Autodesk Inventor part; units mm, degrees
ref_plane "YZ Plane" through (0, 0, 0) normal (1, 0, 0) x (0, 1, 0)
ref_plane "XZ Plane" through (0, 0, 0) normal (0, 1, 0) x (-1, 0, 0)
ref_plane "XY Plane" through (0, 0, 0) normal (0, 0, 1) x (1, 0, 0)
sketch "Sketch1" plane through (0, 0, 0) normal (0, 0, 1) x (1, 0, 0)
  line L0 (0, 0) -> (25, 0)
  line L1 (25, 0) -> (25, 25)
  line L2 (25, 25) -> (0, 25)
  line L3 (0, 25) -> (0, 0)
  dimension "d0" = 25
  dimension "d1" = 25
extrude "Extrusion1" add sketch "Sketch1" along normal blind 2
sketch "Sketch2" plane through (0, 0, 2) normal (0, 0, 1) x (1, 0, 0)
  line L0 (0, 0) -> (0, 25)
  line L1 (0, 25) -> (25, 25)
  line L2 (2.5, 2.5) -> (22.5, 2.5)
  line L3 (22.5, 2.5) -> (22.5, 22.5)
  line L4 (22.5, 22.5) -> (2.5, 22.5)
  line L5 (2.5, 22.5) -> (2.5, 2.5)
  dimension "d4" = 20
  dimension "d5" = 20
  dimension "d6" = 2.5
  dimension "d7" = 2.5
extrude "Extrusion2" add sketch "Sketch2" along normal blind 3
sketch "Sketch3" plane through (0, 0, 0) normal (0, 0, -1) x (-1, 0, 0)
  line L0 (-25, 25) -> (0, 25)
  line L1 (-25, 0) -> (-25, 25)
  line L2 (-23.5, 23.5) -> (-1.5, 23.5)
  line L3 (-1.5, 23.5) -> (-1.5, 1.5)
  line L4 (-1.5, 1.5) -> (-23.5, 1.5)
  line L5 (-23.5, 1.5) -> (-23.5, 23.5)
  dimension "d10" = 22
  dimension "d11" = 22
  dimension "d12" = 1.5
  dimension "d13" = 1.5
extrude "Extrusion3" add sketch "Sketch3" along normal blind 3
properties part number "antena_gps"
Could you check a few things on this model? Use its own coordinates, in mm. A direction names the side the tool comes from. Round coordinates to 2 decimals unless told otherwise and drop trailing zeros. Write each loop counter-clockwise with the first axis right and the second up, starting at its lowest first coordinate (ties: lowest second). Pieces come first, ordered by that corner, then holes. Notation, with made-up numbers: (64, 74) - (79, 74) arc R18 cw to (79, 100) - close; hole circle Ø11 at (31.5, -21.5). An arc over 180 degrees is marked (long way). Use a Markdown table: item, result.
Q1. For pin 1 (1.5 mm diameter, centred on x = 9, z = 3.5, fed in from -Y); pin 2 (2.5 mm diameter, centred on x = 10.5, z = -1.5, fed in from +Y); pin 3 (1.5 mm diameter, centred on y = 12, z = -2, fed in from +X), each with a flat end and sliding along its axis, tell me the tip position at first contact or that it passes through.
Output values:
| item | result |
|---|---|
| pin 1 | y = 2.5 |
| pin 2 | y = 23.5 |
| pin 3 | x = 23.5 |
Q2. I want a section at C-C (z = 2.75). List the corners of the cut face in (x, y) for me.
Output values:
| item | result |
|---|---|
| outline | (2.5, 2.5) - (22.5, 2.5) - (22.5, 22.5) - (2.5, 22.5) - close |
Q3. For faces 1 (the flat face through (13, 22.5, 3)), 2 (the flat face through (23.5, 12, -1)), 3 (the flat face through (12, 1.5, -1)), 4 (the flat face through (12, 2.5, 3)), 5 (the flat face through (1.5, 13, -1)), which set-ups out of +Z, -Z, +X, -X, +Y, -Y let a thin tool reach every point of the face, with its end or its side?
Output values:
| item | result |
|---|---|
| face 1 | +Z, +X, -X, +Y |
| face 2 | -Z, +X, +Y, -Y |
| face 3 | -Z, +X, -X, -Y |
| face 4 | +Z, +X, -X, -Y |
| face 5 | -Z, -X, +Y, -Y |
Q4. I want a section at A-A (y = 10). List the corners of the cut face in (x, z) for me, plus the area to 3 significant figures.
Output values:
| item | result |
|---|---|
| outline | (0, 0) - (1.5, 0) - (1.5, -3) - (23.5, -3) - (23.5, 0) - (25, 0) - (25, 2) - (22.5, 2) - (22.5, 5) - (2.5, 5) - (2.5, 2) - (0, 2) - close |
| area | 176 mm2 |
Q5. Please list where these lines run through material, in increasing order: L1, parallel to Z at x = 2, y = 8.25; L2, parallel to Y at x = 11.75, z = 4.25; L3, parallel to X at y = 5, z = -1.5.
Output values:
| item | result |
|---|---|
| L1 | -3 to 2 |
| L2 | 2.5 to 22.5 |
| L3 | 1.5 to 23.5 |
Q6. I want a section at D-D (z = -2). List the corners of the cut face in (x, y) for me, plus the area to 3 significant figures.
Output values:
| item | result |
|---|---|
| outline | (1.5, 1.5) - (23.5, 1.5) - (23.5, 23.5) - (1.5, 23.5) - close |
| area | 484 mm2 |
